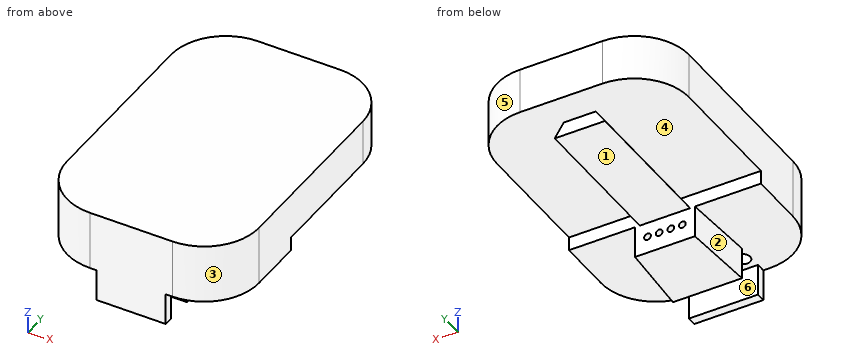
```python
from build123d import *

# Parameters (mm, degrees)
SKETCH_2_W           = 42
SKETCH_2_H           = 63
EXTRUDE_1_DEPTH      = 10
SKETCH_3_W           = 42
SKETCH_3_H           = 24
EXTRUDE_2_DEPTH      = 10
EXTRUDE_3_DEPTH      = 32
SKETCH_5_R           = 0.74
CUT_EXTRUDE_1_DEPTH  = 10
CUT_EXTRUDE_2_DEPTH  = 7
SKETCH_8_R           = 1.6
CUT_EXTRUDE_4_DEPTH  = 3
FILLET_6_R           = 12
CUT_EXTRUDE_21_DEPTH = 7


with BuildPart() as part:
    # Sketch 2 → Extrude 1 (new body)
    with BuildSketch(Plane.XY):
        Rectangle(SKETCH_2_W, SKETCH_2_H)
    extrude(amount=EXTRUDE_1_DEPTH)

    # Sketch 3 → Extrude 2 (add)
    with BuildSketch(Plane(origin=(0, 0, 0), x_dir=(-1, 0, 0), z_dir=(0, 0, -1))):
        with Locations((0, -19.5)):
            Rectangle(SKETCH_3_W, SKETCH_3_H)
    extrude(amount=EXTRUDE_2_DEPTH)

    # Sketch 4 → Extrude 3 (add)
    with BuildSketch(Plane(origin=(0, -7.5, 0), x_dir=(1, 0, 0), z_dir=(0, 1, 0))):
        Polygon((3.5, 0), (5.5, 3), (-5.5, 3), (-3.5, 0), align=None)
    extrude(amount=EXTRUDE_3_DEPTH)

    # Sketch 5 → Cut-Extrude 1 (cut)
    with BuildSketch(Plane(origin=(0, -7.5, 0), x_dir=(1, 0, 0), z_dir=(0, 1, 0))):
        with Locations(Location((-3.81, 6.25, 0), (0, 0, 270))):
            Circle(SKETCH_5_R)
        with Locations(Location((-1.27, 6.25, 0), (0, 0, 270))):
            Circle(SKETCH_5_R)
        with Locations(Location((1.27, 6.25, 0), (0, 0, 270))):
            Circle(SKETCH_5_R)
        with Locations(Location((3.81, 6.25, 0), (0, 0, 270))):
            Circle(SKETCH_5_R)
    extrude(amount=-CUT_EXTRUDE_1_DEPTH, mode=Mode.SUBTRACT)

    # Sketch 6 → Cut-Extrude 2 (cut)
    with BuildSketch(Plane(origin=(0, 0, -10), x_dir=(-1, 0, 0), z_dir=(0, 0, -1))):
        with BuildLine():
            Line((-9.55, -7.5), (-21, -7.5))
            Line((-21, -7.5), (-21, -17.5))
            Line((-21, -17.5), (-19, -17.5))
            Line((-19, -17.5), (-19, -21.5))
            ThreePointArc((-19, -21.5), (-16.656854249, -27.156854249), (-11, -29.5))
            Line((-11, -29.5), (11, -29.5))
            ThreePointArc((11, -29.5), (16.656854249, -27.156854249), (19, -21.5))
            Line((19, -21.5), (19, -17.5))
            Line((19, -17.5), (21, -17.5))
            Line((21, -17.5), (21, -7.5))
            Line((21, -7.5), (9.55, -7.5))
            Line((9.55, -7.5), (9.55, -19.5))
            ThreePointArc((9.55, -19.5), (12.378427125, -20.671572875), (13.55, -23.5))
            ThreePointArc((13.55, -23.5), (11.55, -25.5), (9.55, -23.5))
            Line((9.55, -23.5), (-9.55, -23.5))
            ThreePointArc((-9.55, -23.5), (-11.55, -25.5), (-13.55, -23.5))
            ThreePointArc((-13.55, -23.5), (-12.378427125, -20.671572875), (-9.55, -19.5))
            Line((-9.55, -19.5), (-9.55, -7.5))
        make_face()
    extrude(amount=-CUT_EXTRUDE_2_DEPTH, mode=Mode.SUBTRACT)

    # Sketch 8 → Cut-Extrude 4 (cut)
    with BuildSketch(Plane(origin=(0, 0, -3), x_dir=(-1, 0, 0), z_dir=(0, 0, -1))):
        with Locations((-6, -26.5)):
            Circle(SKETCH_8_R)
        with Locations((6, -26.5)):
            Circle(SKETCH_8_R)
    extrude(amount=-CUT_EXTRUDE_4_DEPTH, mode=Mode.SUBTRACT)

    # Fillet 6
    fillet_6_edges = [part.edges().sort_by_distance(p)[0] for p in [
        (21, -31.5, 0),
        (-21, -31.5, 0),
        (-21, 31.5, 5),
        (21, 31.5, 5),
    ]]
    fillet(fillet_6_edges, radius=FILLET_6_R)

    # Sketch 43 → Cut-Extrude 21 (cut)
    with BuildSketch(Plane(origin=(0, 0, -10), x_dir=(-1, 0, 0), z_dir=(0, 0, -1))):
        Polygon((-7.55, -7.5), (-21, -7.5), (-21, -31.5), (-7.55, -31.5), (-7.55, -23.5), (-6.55, -7.5), align=None)
        Polygon((21, -7.5), (21, -31.5), (7.55, -31.5), (7.55, -23.5), (6.55, -7.5), (7.55, -7.5), align=None)
    extrude(amount=-CUT_EXTRUDE_21_DEPTH, mode=Mode.SUBTRACT)


solid = part.part
```
Geometry: final body of the model. Coordinates: model frame, mm. Face numbers are marked on the shaded views. A direction names the side the tool comes from. Round coordinates to 2 decimals unless told otherwise and drop trailing zeros. Order: outer loops, then holes, each group sorted by start corner. A loop starts at its lowest first (then second) coordinate and runs counter-clockwise, first axis right, second up. Notation, with made-up numbers: M 41,-25.5 L 58,-25.5 A16 ccw 58,-14.5 Z; hole C 74,47.25 d6. An arc over 180 degrees is marked long. Use one line per item in the form item = value. Start each with the question number.
Q1. Access query for the marked faces 1, 2 and 3. Directions: +Z, -Z, +X, -X, +Y, -Y. A direction counts if a zero-diameter tool reaches every point of the face in a straight line with its end or side. Return the directions, or none.
Q2. Pin query (flat end, axial travel): pin 1 Ø1.6 at (y, z) = (-30.5, -7.5) entering from +X; pin 2 Ø4 at (x, z) = (-13, -1) entering from -Y; pin 3 Ø5.5 at (x, y) = (0, 8) entering from -Z. Return the tip coordinate at first contact, or that it passes through.
Q3. Material intervals for line 1 (X direction, y = -13, z = -6.25); line 2 (Y direction, x = 3.5, z = -7.5); line 3 (Y direction, x = 6, z = -0.5), sorted ascending. Write a range as [from, to].
Q4. Mould query, pull axis Y, two halves, no side actions, for the marked faces 4, 5 and 6. Classes: +Y half, -Y half, draft (parallel to the pull), parting line (faces both ways), or undercut.
Q5. Cut plane A-A (z = -6.25). Return loops of the section in (x, y), and give its area (3 significant figures).
Q6. Cut plane C-C (x = -1.27). Return loops of the section in (y, z).
Q7. Cut plane B-B (z = -1.5). Return loops of the section in (x, y).
Q8. Cut plane D-D (y = 8). Return loops of the section in (x, z), and give its area (3 significant figures).
Geometry results:
q1.face_1 = -Z, +X, -X, +Y
q1.face_2 = -Z, -X, +Y
q1.face_3 = +Z, -Z, +X, -Y
q2.pin_1 = 7.55
q2.pin_2 = -31.33
q2.pin_3 = -3
q3.line_1 = [-6.89, -4.55], [-3.07, -2.01], [-0.53, 0.53], [2.01, 3.07], [4.55, 6.89]
q3.line_2 = [-31.5, -29.5], [-23.5, -7.5]
q3.line_3 = [-31.5, -28.1], [-24.9, -7.5]
q4.face_4 = draft
q4.face_5 = +Y half
q4.face_6 = undercut
q5.outline = M -7.55,-31.5 L 7.55,-31.5 L 7.55,-29.5 L -7.55,-29.5 Z; M -7.55,-23.5 L 7.55,-23.5 L 6.55,-7.5 L 4.55,-7.5 L 4.55,-17.5 L 3.07,-17.5 L 3.07,-7.5 L 2.01,-7.5 L 2.01,-17.5 L 0.53,-17.5 L 0.53,-7.5 L -0.53,-7.5 L -0.53,-17.5 L -2.01,-17.5 L -2.01,-7.5 L -3.07,-7.5 L -3.07,-17.5 L -4.55,-17.5 L -4.55,-7.5 L -6.55,-7.5 Z
q5.area = 197 mm^2
q6.outline = M -31.5,-10 L -29.5,-10 L -29.5,-3 L -23.5,-3 L -23.5,-10 L -7.5,-10 L -7.5,-6.99 L -17.5,-6.99 L -17.5,-5.51 L -7.5,-5.51 L -7.5,-3 L 24.5,-3 L 24.5,0 L 31.5,0 L 31.5,10 L -31.5,10 Z
q7.outline = M -21,-19.5 A12 ccw -9,-31.5 L 9,-31.5 A12 ccw 21,-19.5 L 21,-7.5 L 4.5,-7.5 L 4.5,24.5 L -4.5,24.5 L -4.5,-7.5 L -21,-7.5 Z; hole C -6,-26.5 d3.2; hole C 6,-26.5 d3.2
q8.outline = M -21,0 L -3.5,0 L -5.5,-3 L 5.5,-3 L 3.5,0 L 21,0 L 21,10 L -21,10 Z
q8.area = 447 mm^2
